Study the drawing (mm; zero at the part's minimum x, y, z) and answer. Coordinates: 2 decimals unless noted, no trailing zeros. Order: outer loops, then holes, each group sorted by start corner. A loop starts at its lowest first (then second) coordinate and runs counter-clockwise, first axis right, second up.
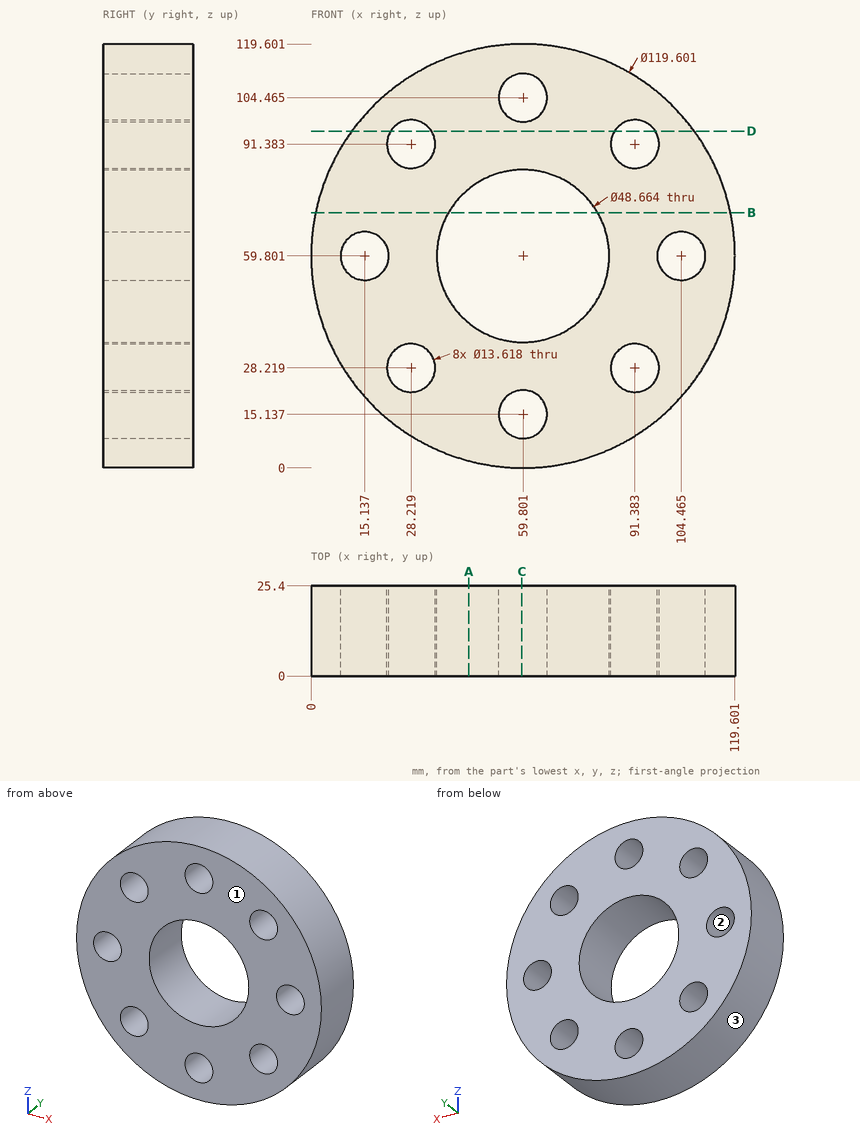
(1) Given pin 1 Ø1.5 at (y, z) = (9, 88.5) entering from -X; pin 2 Ø5 at (y, z) = (6.5, 103.5) entering from -X (1 decimal); pin 3 Ø5 at (x, y) = (37.5, 10) entering from +Z, each flat-ended and moving along its own axis, determine where each tip first touches the part or whether it passes through.
(2) Find section A-A on x = 44.5. Determine the outline of the cut face in (y, z).
(3) Find section B-B on z = 72. Determine the outline of the cut face in (x, y).
(4) Find section C-C on x = 59.5. Determine the outline of the cut face in (y, z) (1 decimal).
(5) Find the intervals of material crossed by probe 1 along X at (y, z) = (22.5, 59) (1 decimal); probe 2 along X at (y, z) = (2.5, 30.5) (1 decimal); probe 3 along X at (y, z) = (16.5, 57) (1 decimal), in increasing order.
(6) The mould has two halves that part along X. Classify the marked faces 1, 2 and 3: pulls with the +X half, pulls with the -X half, needs draft (parallel to the pull), parting line crosses it, or undercut.
(7) Find section D-D on z = 95. Count the separate pieces of the cut face and the enclosed holes in it, then the cut area to 3 significant figures.
Resolved:
1. pin 1: stops at x = 6.93
1. pin 2: stops at x = 16.5
1. pin 3: stops at z = 116.23
2. outline: (0, 1.99) - (25.4, 1.99) - (25.4, 40.88) - (0, 40.88) - close; (0, 78.72) - (25.4, 78.72) - (25.4, 117.61) - (0, 117.61) - close
3. outline: (1.26, 0) - (38.75, 0) - (38.75, 25.4) - (1.26, 25.4) - close; (80.85, 0) - (118.34, 0) - (118.34, 25.4) - (80.85, 25.4) - close
4. outline: (0, 0) - (25.4, 0) - (25.4, 8.3) - (0, 8.3) - close; (0, 21.9) - (25.4, 21.9) - (25.4, 35.5) - (0, 35.5) - close; (0, 84.1) - (25.4, 84.1) - (25.4, 97.7) - (0, 97.7) - close; (0, 111.3) - (25.4, 111.3) - (25.4, 119.6) - (0, 119.6) - close
5. probe 1: x = 0 to 8.4, 21.9 to 35.5, 84.1 to 97.7, 111.2 to 119.6
5. probe 2: x = 7.7 to 21.8, 34.6 to 85, 97.8 to 111.9
5. probe 3: x = 0.1 to 8.9, 21.3 to 35.6, 84 to 98.3, 110.7 to 119.5
6. face 1: needs draft
6. face 2: undercut
6. face 3: parting line crosses it
7. separate pieces: 3
7. enclosed holes: 0
7. area: 1,870 mm2
